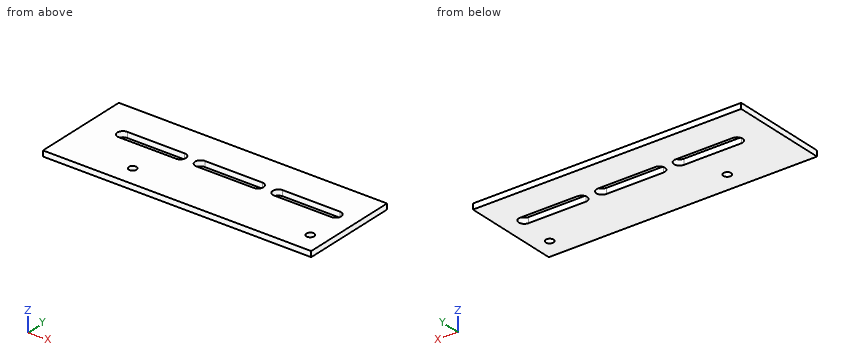
```python
from build123d import *

# Parameters (mm, degrees)
LID_RISER_WITH_VENTS_PROFILE_W = 145
LID_RISER_WITH_VENTS_PROFILE_H = 53
LID_RISER_WITH_VENTS_PROFILE_R = 2.1
LID_RISER_WITH_VENTS_DEPTH     = 3


with BuildPart() as part:
    # Lid riser with vents profile → Lid riser with vents (new body)
    with BuildSketch(Plane.XY):
        with Locations((-18.5, 76.5)):
            Rectangle(LID_RISER_WITH_VENTS_PROFILE_W, LID_RISER_WITH_VENTS_PROFILE_H)
        with Locations((-51, 61)):
            Circle(LID_RISER_WITH_VENTS_PROFILE_R, mode=Mode.SUBTRACT)
        with Locations((45, 61)):
            Circle(LID_RISER_WITH_VENTS_PROFILE_R, mode=Mode.SUBTRACT)
        with BuildLine():
            Line((-72.5, 79), (-41.5, 79))
            ThreePointArc((-41.5, 79), (-38.5, 82), (-41.5, 85))
            Line((-41.5, 85), (-72.5, 85))
            ThreePointArc((-72.5, 85), (-75.5, 82), (-72.5, 79))
        make_face(mode=Mode.SUBTRACT)
        with BuildLine():
            Line((-30.5, 79), (0.5, 79))
            ThreePointArc((0.5, 79), (3.5, 82), (0.5, 85))
            Line((0.5, 85), (-30.5, 85))
            ThreePointArc((-30.5, 85), (-33.5, 82), (-30.5, 79))
        make_face(mode=Mode.SUBTRACT)
        with BuildLine():
            Line((11.5, 79), (42.5, 79))
            ThreePointArc((42.5, 79), (45.5, 82), (42.5, 85))
            Line((42.5, 85), (11.5, 85))
            ThreePointArc((11.5, 85), (8.5, 82), (11.5, 79))
        make_face(mode=Mode.SUBTRACT)
    extrude(amount=LID_RISER_WITH_VENTS_DEPTH)


solid = part.part
```
Can you work these out from the model? Positions are in its coordinate system, mm. Give positions to 0.01 mm unless a question says otherwise; leave off trailing zeros. Write each loop counter-clockwise with the first axis right and the second up, starting at its lowest first coordinate (ties: lowest second). Pieces come first, ordered by that corner, then holes. Notation, with made-up numbers: (-7, -24.5) - (15, -24.5) arc R14 cw to (15, 0.5) - close; hole circle Ø11 at (67, 85). An arc over 180 degrees is marked (long way). Write item = value, one per line. Start each with the question number.
1. Imagine slicing it at D-D (x = 21). Please give me the cut outline in (y, z), and give its area (3 significant figures).
2. Imagine slicing it at B-B (y = 61). Please give me the cut outline in (x, z), and give its area (3 significant figures).
3. Imagine slicing it at C-C (z = 2.45). Please give me the cut outline in (x, y), and give its area (3 significant figures).
4. Imagine slicing it at A-A (x = -51). Please give me the cut outline in (y, z).
5. For pin 1 (2.5 mm diameter, centred on x = -51, y = 61, fed in from -Z), with a flat end and sliding along its axis, tell me the tip position at first contact or that it passes through.
6. Please list where these lines run through material, in increasing order: line 1 (Y direction, x = -51, z = 1.75); line 2 (Y direction, x = -64, z = 1.5); line 3 (X direction, y = 60.5, z = 1.3).
Worked answers:
q1.outline = (50, 0) - (79, 0) - (79, 3) - (50, 3) - close; (85, 0) - (103, 0) - (103, 3) - (85, 3) - close
q1.area = 141 mm2
q2.outline = (-91, 0) - (-53.1, 0) - (-53.1, 3) - (-91, 3) - close; (-48.9, 0) - (42.9, 0) - (42.9, 3) - (-48.9, 3) - close; (47.1, 0) - (54, 0) - (54, 3) - (47.1, 3) - close
q2.area = 410 mm2
q3.outline = (-91, 50) - (54, 50) - (54, 103) - (-91, 103) - close; hole (-72.5, 79) - (-41.5, 79) arc R3 ccw to (-41.5, 85) - (-72.5, 85) arc R3 ccw to start; hole circle Ø4.2 at (-51, 61); hole (-30.5, 79) - (0.5, 79) arc R3 ccw to (0.5, 85) - (-30.5, 85) arc R3 ccw to start; hole (11.5, 79) - (42.5, 79) arc R3 ccw to (42.5, 85) - (11.5, 85) arc R3 ccw to start; hole circle Ø4.2 at (45, 61)
q3.area = 7,010 mm2
q4.outline = (50, 0) - (58.9, 0) - (58.9, 3) - (50, 3) - close; (63.1, 0) - (79, 0) - (79, 3) - (63.1, 3) - close; (85, 0) - (103, 0) - (103, 3) - (85, 3) - close
q5.pin_1 = through
q6.line_1 = 50 to 58.9, 63.1 to 79, 85 to 103
q6.line_2 = 50 to 79, 85 to 103
q6.line_3 = -91 to -53.04, -48.96 to 42.96, 47.04 to 54
